```python
from build123d import *

# Parameters (mm, degrees)
EXTRUDE_1_DEPTH            = 90
HOLE_WIZARD_M52_AT_2_COUNT = 2
HOLE_WIZARD_M52_AT_2_PITCH = 63
HOLE_WIZARD_M52_AT_3_COUNT = 2
HOLE_WIZARD_M52_AT_3_PITCH = 93
HOLE_WIZARD_M52_AT_4_COUNT = 2
HOLE_WIZARD_M52_AT_4_PITCH = 156


with BuildPart() as part:
    # Эскиз1 → Бобышка-Вытянуть1 (new body, symmetric)
    with BuildSketch(Plane.XY):
        Polygon((4, 0), (-4, 0), (-4, -1.9), (-7.9, -1.9), (-7.9, -3.4), (-4, -6), (4, -6), (7.9, -3.4), (7.9, -1.9), (4, -1.9), align=None)
    extrude(amount=EXTRUDE_1_DEPTH, both=True)

    # Эскиз6 → Отверстие обработанное метчиком M52 (revolve, cut)
    with BuildSketch(Plane(origin=(0, 0, -78), x_dir=(0, 0, 1), z_dir=(1, 0, 0))):
        Polygon((0, 0), (0, 6), (2.525, 6), (2.1, 5.575), (2.1, 0.425), (2.525, 0), align=None)
    hole_wizard_m52 = revolve(axis=Axis((0, 6.35, -78), (0, -1, 0)), mode=Mode.SUBTRACT)

    # Отверстие обработанное метчиком M52 at 2: Отверстие обработанное метчиком M52 ×2
    with Locations(*[(0, 0, i * HOLE_WIZARD_M52_AT_2_PITCH) for i in range(1, HOLE_WIZARD_M52_AT_2_COUNT)]):
        add(hole_wizard_m52, mode=Mode.SUBTRACT)

    # Отверстие обработанное метчиком M52 at 3: Отверстие обработанное метчиком M52 ×2
    with Locations(*[(0, 0, i * HOLE_WIZARD_M52_AT_3_PITCH) for i in range(1, HOLE_WIZARD_M52_AT_3_COUNT)]):
        add(hole_wizard_m52, mode=Mode.SUBTRACT)

    # Отверстие обработанное метчиком M52 at 4: Отверстие обработанное метчиком M52 ×2
    with Locations(*[(0, 0, i * HOLE_WIZARD_M52_AT_4_PITCH) for i in range(1, HOLE_WIZARD_M52_AT_4_COUNT)]):
        add(hole_wizard_m52, mode=Mode.SUBTRACT)


solid = part.part
```
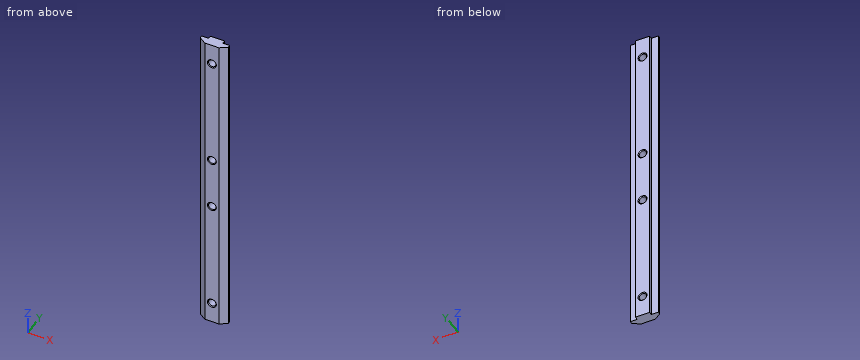
Can you work these out from the model? Positions are in its coordinate system, mm. Give positions to 0.01 mm unless a question says otherwise; leave off trailing zeros. Order: outer loops, then holes, each group sorted by start corner. A loop starts at its lowest first (then second) coordinate and runs counter-clockwise, first axis right, second up. Notation, with made-up numbers: (10.25, 71) - (53.25, 71) arc R5 ccw to (53.25, 77) - close; hole circle Ø7 at (-4.75, 46). An arc over 180 degrees is marked (long way). Use a Markdown table: item, result. Add a question column.
Q1. If we section it at B-B on y = -4.4: Write out the boundary of the cut face in (x, z).
Q2. I'm going to push flat-ended pins straight in: pin 1 (1.2 mm diameter, centred on x = 6, z = 41.5, fed in from +Y); pin 2 (1.5 mm diameter, centred on y = -1, z = 33.5, fed in from -X); pin 3 (1.5 mm diameter, centred on y = -1, z = 20.5, fed in from +X); pin 4 (3.5 mm diameter, centred on x = 0, z = 15, fed in from -Y). Where does each tip first touch, or does it pass through?
Q3. Please list where these lines run through material, in increasing order: line 1 along Z through (x, y) = (0, -4.3); line 2 along X through (y, z) = (-2.55, -78); line 3 along Z through (x, y) = (-1, -3.7).
Q4. If we section it at C-C on x = 0: Count the separate pieces of the cut face and the enclosed holes in it, plus the area to 3 significant figures.
Q5. If we section it at A-A on z = -15: Write out the boundary of the cut face in (x, y) (3 decimals).
Answers follow:
| question | item | result |
|---|---|---|
| 1 | outline | (-6.4, -90) - (6.4, -90) - (6.4, 90) - (-6.4, 90) - close; hole circle Ø4.2 at (0, -78); hole circle Ø4.2 at (0, -15); hole circle Ø4.2 at (0, 15); hole circle Ø4.2 at (0, 78) |
| 2 | pin 1 | stops at y = -1.9 |
| 2 | pin 2 | stops at x = -4 |
| 2 | pin 3 | stops at x = 4 |
| 2 | pin 4 | passes through |
| 3 | line 1 | z = -90 to -80.1, -75.9 to -17.1, -12.9 to 12.9, 17.1 to 75.9, 80.1 to 90 |
| 3 | line 2 | x = -7.9 to -2.1, 2.1 to 7.9 |
| 3 | line 3 | z = -90 to -79.85, -76.15 to -16.85, -13.15 to 13.15, 16.85 to 76.15, 79.85 to 90 |
| 4 | separate pieces | 5 |
| 4 | enclosed holes | 0 |
| 4 | area | 978 mm^2 |
| 5 | outline | (-7.9, -3.4) - (-4, -6) - (-2.525, -6) - (-2.1, -5.575) - (-2.1, -0.425) - (-2.525, 0) - (-4, 0) - (-4, -1.9) - (-7.9, -1.9) - close; (2.1, -5.575) - (2.525, -6) - (4, -6) - (7.9, -3.4) - (7.9, -1.9) - (4, -1.9) - (4, 0) - (2.525, 0) - (2.1, -0.425) - close |
